Input: part model. Units: mm. Frame: model coordinates. Face numbers are marked on the shaded views. A direction names the side the tool comes from. Round coordinates to 2 decimals unless told otherwise and drop trailing zeros. Loops run counter-clockwise (first coordinate to the right, second up) from the corner with the lowest first, then second, coordinate; pieces in that order, holes last. Notation, with made-up numbers: M 46.5,-25 L 66.5,-25 A17 cw 66.5,-15 Z; hole C 3,-35 d8. An arc over 180 degrees is marked long. Put each result on its own line as item: value. Start each with the question number.
1) Section C-C on y = -44. Output: boundary loops of the cut face in (x, z).
2) Line query: probe 1 along Y at (x, z) = (0, 2.6); probe 2 along Z at (x, y) = (2, 5.5); probe 3 along Y at (x, z) = (18, 2). Output: solid intervals per line, ascending.
3) Section A-A on z = 7. Output: boundary loops of the cut face in (x, y), plus the area to 3 significant figures.
4) Pin query (flat end, axial travel): pin 1 (5 mm diameter, centred on x = -4.5, y = 12, fed in from +Z); pin 2 (8 mm diameter, centred on y = -24, z = 8.5, fed in from -X); pin 3 (1 mm diameter, centred on x = -15, z = 6.5, fed in from -Y); pin 4 (3 mm diameter, centred on x = -32.5, z = 5.5, fed in from -Y). Return the tip coordinate at first contact, or that it passes through.
5) Reachability of the marked faces 1 and 2 from +Z, -Z, +X, -X, +Y, -Y: full face, straight path, thin tool, end or side. Return the list, or none.
6) Section D-D on x = -33. Output: boundary loops of the cut face in (y, z), plus the area to 3 significant figures.
7) Section B-B on y = 0. Output: boundary loops of the cut face in (x, z), plus the area to 4 significant figures.
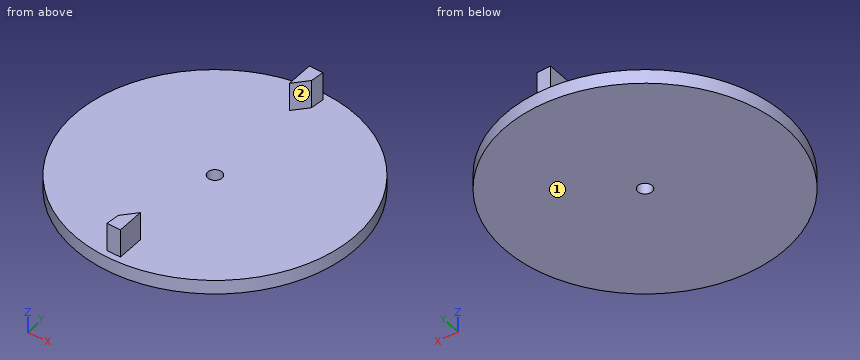
from build123d import *

# Parameters (mm, degrees)
F0_R     = 50
F0_R_2   = 2.55
F1_DEPTH = 5
F3_DEPTH = 10


with BuildPart() as f1:
    # F0 (on Top) → F1 (new body)
    with BuildSketch(Plane.XY):
        Circle(F0_R)
        Circle(F0_R_2, mode=Mode.SUBTRACT)
    extrude(amount=F1_DEPTH)

    # F2 (on face) → F3 (join)
    with BuildSketch(Plane.XY.offset(5)):
        Polygon((5.046888, 47.231122), (0.046888, 47.495013), (0.046888, 37.495013), (4.520572, 42.2589), align=None)
        Polygon((-5, -47.361098), (0, -47.624989), (0, -37.624989), (-4.473684, -42.388876), align=None)
    extrude(amount=F3_DEPTH)


solid = f1.part
Geometry results:
1. outline: M -23.75,0 L 23.75,0 L 23.75,5 L 0,5 L 0,15 L -4.64,15 L -4.64,5 L -23.75,5 Z
2. probe 1: y = -50 to -2.55, 2.55 to 50
2. probe 2: z = 0 to 5
2. probe 3: y = -46.65 to 46.65
3. outline: M -5,-47.36 L 0,-47.62 L 0,-37.62 L -4.47,-42.39 Z; M 0.05,37.5 L 4.52,42.26 L 5.05,47.23 L 0.05,47.5 Z
3. area: 69.7 mm²
4. pin 1: stops at z = 5
4. pin 2: stops at x = -44.87
4. pin 3: passes through
4. pin 4: stops at y = -39.16
5. face 1: -Z, +X, -X, +Y, -Y
5. face 2: +Z, +X, -Y
6. outline: M -37.56,0 L 37.56,0 L 37.56,5 L -37.56,5 Z
6. area: 376 mm²
7. outline: M -50,0 L -2.55,0 L -2.55,5 L -50,5 Z; M 2.55,0 L 50,0 L 50,5 L 2.55,5 Z
7. area: 474.5 mm²
